from build123d import *

# Parameters (mm, degrees)
F0_R           = 12.5
F1_DEPTH       = 15
F3_DEPTH       = 8
F5_DEPTH       = 9
F6_R           = 1.4
F7_DEPTH       = 5.9
F9_W           = 6
F9_H           = 6
F10_DEPTH      = 3
F11_R          = 1.4
F12_DEPTH      = 12.5010001
F12_DEPTH_BACK = 12.5010001


with BuildPart() as f1:
    # F0 (on Top) → F1 (new body)
    with BuildSketch(Plane.XY):
        Circle(F0_R)
    extrude(amount=F1_DEPTH)

    # F2 (on face) → F3 (cut)
    with BuildSketch(Plane(origin=(0, 0, 0), x_dir=(1, 0, 0), z_dir=(0, 0, -1))):
        with BuildLine():
            Line((-3.8729833462, 1), (-12.5, 1))
            Line((-12.5, 1), (-12.5, -1))
            Line((-12.5, -1), (-3.8729833462, -1))
            ThreePointArc((-3.8729833462, -1), (-2.8284271247, -2.8284271247), (-1, -3.8729833462))
            Line((-1, -3.8729833462), (-1, -12.5))
            Line((-1, -12.5), (1, -12.5))
            Line((1, -12.5), (1, -3.8729833462))
            ThreePointArc((1, -3.8729833462), (2.8284271247, -2.8284271247), (3.8729833462, -1))
            Line((3.8729833462, -1), (12.5, -1))
            Line((12.5, -1), (12.5, 1))
            Line((12.5, 1), (3.8729833462, 1))
            ThreePointArc((3.8729833462, 1), (2.8284271247, 2.8284271247), (1, 3.8729833462))
            Line((1, 3.8729833462), (1, 12.5))
            Line((1, 12.5), (-1, 12.5))
            Line((-1, 12.5), (-1, 3.8729833462))
            ThreePointArc((-1, 3.8729833462), (-2.8284271247, 2.8284271247), (-3.8729833462, 1))
        make_face()
    extrude(amount=-F3_DEPTH, mode=Mode.SUBTRACT)

    # F4 (on face) → F5 (cut)
    with BuildSketch(Plane.XY.offset(15)):
        Polygon((3.8105117767, 6.6), (-3.8105117767, 6.6), (-7.6210235533, 0), (-3.8105117767, -6.6), (3.8105117767, -6.6), (7.6210235533, 0), align=None)
    extrude(amount=-F5_DEPTH, mode=Mode.SUBTRACT)

    # F6 (on face) → F7 (cut, through all)
    with BuildSketch(Plane(origin=(-5.715767665, 3.3, 0), x_dir=(0.5, 0.8660254038, 0), z_dir=(0.8660254038, -0.5, 0))):
        with Locations((0, 12.8758029834)):
            Circle(F6_R)
    extrude(amount=-F7_DEPTH, mode=Mode.SUBTRACT)

    # F9 (on offset) → F10 (cut)
    with BuildSketch(Plane(origin=(-7.0148057707, 4.05, 0), x_dir=(0.5, 0.8660254038, 0), z_dir=(0.8660254038, -0.5, 0))):
        with Locations((0, 12.8758029834)):
            Rectangle(F9_W, F9_H)
    extrude(amount=-F10_DEPTH, mode=Mode.SUBTRACT)

    # F11 (on Right) → F12 (cut, two sides)
    with BuildSketch(Plane.YZ) as f12_sk:
        with Locations((6.542795848, 2.5)):
            Circle(F11_R)
        with Locations((-6.542795848, 2.5)):
            Circle(F11_R)
    extrude(amount=-F12_DEPTH, mode=Mode.SUBTRACT)
    extrude(f12_sk.sketch, amount=F12_DEPTH_BACK, mode=Mode.SUBTRACT)


solid = f1.part
For this review, take the finished solid that the model builds, in its own axes (mm). A direction names the side the tool comes from. Give positions to 0.01 mm unless a question says otherwise; leave off trailing zeros. Loops run counter-clockwise (first coordinate to the right, second up) from the corner with the lowest first, then second, coordinate; pieces in that order, holes last. Notation, with made-up numbers: M 19.25,66 L 65.25,66 A8 cw 65.25,75 Z; hole C -32.5,-16.75 d11. An arc over 180 degrees is marked long. Answer as a JSON object with one key per item and string values. Group by question number.
Q1. Add section C-C on y = -2.5. Give the boundary of the cut face in (x, z), and give its area (3 significant figures).
Q2. For probe 1 along Y at (x, z) = (5.75, 2.5); probe 2 along Y at (x, z) = (-7.5, 2.5); probe 3 along Z at (x, y) = (3, -4.25), list the stretches that pass through material, from the lowest coordinate up. Write a range as [from, to].
Q3. Mouldability with a two-part tool opening along X and no side actions: class faces 1 (the cylindrical face through (11.923, 3.755, 7.395)), 2 (the flat face through (-9.796, 2.191, 12.402)), 3 (the flat face through (5, -5, 15)) as +X half, -X half, draft (parallel to the pull), parting line (faces both ways), or undercut.
Q4. Insertion check: P1, Ø6, axis at x = -7.5, z = 13.5, coming from the -Y side; P2, Ø6.5, axis at y = 7, z = 5, coming from the -X side; P3, Ø4, axis at y = 8, z = 7, coming from the +X side. Each pin has a flat end and moves straight along its axis. Give the tip position at first contact, or say it passes through.
Q5. Tool access review of faces 4 (the flat face through (8, -1, 4)), 5 (the flat face through (1, 8, 4)), 6 (the cylindrical face through (-2.807, -2.849, 2.958)), 7 (the flat face through (0, -6.6, 11)): name each direction out of +Z, -Z, +X, -X, +Y, -Y from which nothing blocks a thin tool from reaching the whole face with its end or side.
Q6. Add section D-D on z = 1.75. Give the number of separate pieces and of enclosed holes in the cut face, and give its area (3 significant figures).
Q7. Add section B-B on x = -2.75. Give the boundary of the cut face in (y, z), and give its area (3 significant figures).
Q8. Add section A-A on x = 0.5. Give the boundary of the cut face in (y, z), and give its area (3 significant figures).
Checked values:
{
 "1": {"outline": "M -12.25,0 L -3.12,0 L -3.12,6 L -6.18,6 L -6.18,15 L -12.25,15 Z; M 3.12,0 L 12.25,0 L 12.25,15 L 6.18,15 L 6.18,6 L 3.12,6 Z", "area": "219 mm²"},
 "2": {"probe 1": "[-11.1, -7.94], [-5.14, -1], [1, 5.14], [7.94, 11.1]", "probe 2": "[-10, -7.94], [-5.14, -1], [1, 5.14], [7.94, 10]", "probe 3": "[0, 6]"},
 "3": {"face 1": "parting line", "face 2": "undercut", "face 3": "draft"},
 "4": {"P1": "y = -11.66", "P2": "x = -11.92", "P3": "x = 10.97"},
 "5": {"face 4": "-Z, +X, -X", "face 5": "-Z, +Y, -Y", "face 6": "+Z, -Z", "face 7": "+Z"},
 "6": {"separate pieces": "8", "enclosed holes": "0", "area": "281 mm²"},
 "7": {"outline": "M -12.19,0 L -2.9,0 L -2.9,6 L -6.6,6 L -6.6,15 L -12.19,15 Z; M 2.9,0 L 12.19,0 L 12.19,15 L 6.6,15 L 6.6,6 L 2.9,6 Z; hole C -6.54,2.5 d2.8; hole C 6.54,2.5 d2.8", "area": "200 mm²"},
 "8": {"outline": "M -12.49,8 L -6.6,8 L -6.6,15 L -12.49,15 Z; M 6.6,8 L 12.49,8 L 12.49,15 L 6.6,15 Z", "area": "82.5 mm²"}
}
